Read the model definition and answer for the solid it produces. Units are mm, in the model's axes. A direction names the side the tool comes from. Give positions to 0.01 mm unless a question says otherwise; leave off trailing zeros. Loops run counter-clockwise (first coordinate to the right, second up) from the corner with the lowest first, then second, coordinate; pieces in that order, holes last. Notation, with made-up numbers: (60, 54.5) - (80, 54.5) arc R18 cw to (80, 61.5) - close; hole circle Ø4 at (77.25, 15). An arc over 180 degrees is marked (long way). Write each question's results on one line, items separated by ' | '. Start each with the question number.
Q1. Determine the mould class of faces 1 (the cylindrical face through (-0.106, 5.817, -24.136)), 2 (the flat face through (0, 0, 0)), 3 (the flat face through (0, 6, 6.75)) for opening direction Z: +Z half, -Z half, draft (parallel to the pull), parting line (faces both ways), or undercut.
Q2. For faces 4 (the cylindrical face through (-0.41, 3.377, -11.448)), 5 (the flat face through (0, 13, 0)), determine the directions among +Z, -Z, +X, -X, +Y, -Y from which every point of the face is accessible in a straight line to the end or side of a thin tool.
Q3. Given pin 1 (1.5 mm diameter, centred on x = -5, z = -9.5, fed in from -Y); pin 2 (6 mm diameter, centred on x = -4, y = 3, fed in from -Z); pin 3 (8 mm diameter, centred on y = 4, z = -13.5, fed in from +X); pin 4 (6 mm diameter, centred on x = -0.5, z = -18.5, fed in from -Y), each flat-ended and moving along its own axis, determine where each tip first touches the part or whether it passes through.
Q4. Find the intervals of material crossed by line 1 (Z direction, x = 6.25, y = 11.5); line 2 (Z direction, x = -3.5, y = 7); line 3 (Y direction, x = 4.75, z = -6), in increasing order. Write a range as from..to.
Q5. The part is cut by section D-D, the plane x = 0. Write down the section's boundary in (y, z).
Q6. The part is cut by section A-A, the plane y = 12. Write down the section's boundary in (x, z).
Q7. The part is cut by section B-B, the plane x = -5.5. Write down the section's boundary in (y, z).
Q8. The part is cut by section C-C, the plane z = -10. Write down the section's boundary in (x, y).
```python
from build123d import *

# Parameters (mm, degrees)
SKETCH1_W           = 13
SKETCH1_H           = 13.5
BOSS_EXTRUDE1_DEPTH = 13
SKETCH2_R           = 3.15
BOSS_EXTRUDE2_DEPTH = 8.5
SKETCH3_R           = 4
BOSS_EXTRUDE3_DEPTH = 1
CHAMFER1_SIZE       = 0.2


with BuildPart() as part:
    # Sketch1 → Boss-Extrude1 (new body)
    with BuildSketch(Plane(origin=(0, 0, 0), x_dir=(1, 0, 0), z_dir=(0, 1, 0))):
        Rectangle(SKETCH1_W, SKETCH1_H)
    extrude(amount=BOSS_EXTRUDE1_DEPTH)

    # Sketch2 → Boss-Extrude2 (add)
    with BuildSketch(Plane(origin=(0, 0, -6.75), x_dir=(-1, 0, 0), z_dir=(0, 0, -1))):
        with Locations(Location((0, 6.5, 0), (0, 0, 180))):
            Circle(SKETCH2_R)
    extrude(amount=BOSS_EXTRUDE2_DEPTH)

    # Sketch3 → Boss-Extrude3 (add)
    with BuildSketch(Plane(origin=(0, 0, -6.75), x_dir=(-1, 0, 0), z_dir=(0, 0, -1))):
        with Locations(Location((0, 6.5, 0), (0, 0, 180))):
            Circle(SKETCH3_R)
    extrude(amount=BOSS_EXTRUDE3_DEPTH)

    # Sketch4 → Revolve1 (revolve)
    with BuildSketch(Plane(origin=(0, 0, 0), x_dir=(0, 0, -1), z_dir=(1, 0, 0))):
        with BuildLine():
            Line((14.310307379, 6.842020143), (13.865681193, 5.620419736))
            Line((13.865681193, 5.620419736), (17.154605366, 4.423349235))
            Line((17.154605366, 4.423349235), (16.778383208, 3.389687352))
            Line((16.778383208, 3.389687352), (28.242633182, -0.782958397))
            Line((28.242633182, -0.782958397), (28.635956346, 0.297688117))
            ThreePointArc((28.635956346, 0.297688117), (29.283711619, 0.637305625), (29.693868496, 1.2428618))
            Line((29.693868496, 1.2428618), (14.310307379, 6.842020143))
        make_face()
    revolve(axis=Axis((0, 6.5, -15.25), (0, -0.34202014332566943, -0.9396926207859081)))

    # Chamfer1
    chamfer1_edges = [part.edges().sort_by_distance(p)[0] for p in [
        (0, 3.727566183, -29.88432987),
    ]]
    chamfer(chamfer1_edges, length=CHAMFER1_SIZE)


solid = part.part
```
Check sheet entries:
1) face 1: undercut | face 2: draft | face 3: +Z half
2) face 4: none | face 5: +Z, -Z, +X, -X, +Y
3) pin 1: passes through | pin 2: stops at z = -29.73 | pin 3: stops at x = 3.15 | pin 4: stops at y = 1.68
4) line 1: z = -6.75..6.75 | line 2: z = -7.75..6.75 | line 3: y = 0..13
5) outline: (-0.71, -28.05) - (-0.6, -28.31) - (0.3, -28.64) arc R1.5 ccw to (2.65, -29.49) - (3.54, -29.82) - (3.8, -29.7) - (7.9, -18.42) - (6.87, -18.04) - (7.88, -15.25) - (9.65, -15.25) - (9.65, -7.75) - (10.5, -7.75) - (10.5, -6.75) - (13, -6.75) - (13, 6.75) - (0, 6.75) - (0, -6.75) - (2.5, -6.75) - (2.5, -7.75) - (3.35, -7.75) - (3.35, -15.25) - (5.12, -15.25) - (4.42, -17.15) - (3.39, -16.78) - close
6) outline: (-6.5, -6.75) - (6.5, -6.75) - (6.5, 6.75) - (-6.5, 6.75) - close
7) outline: (0, -6.75) - (13, -6.75) - (13, 6.75) - (0, 6.75) - close
8) outline: circle Ø6.3 at (0, 6.5)
